Work out the finished part from the listing and answer in its coordinate system (mm). A direction names the side the tool comes from. Round coordinates to 2 decimals unless told otherwise and drop trailing zeros. Loops run counter-clockwise (first coordinate to the right, second up) from the corner with the lowest first, then second, coordinate; pieces in that order, holes last. Notation, with made-up numbers: (-12.5, 35.5) - (28.5, 35.5) arc R10 ccw to (28.5, 51.5) - close; hole circle Ø7 at (78.25, 37). An arc over 180 degrees is marked (long way). Return JSON: item names as keys, results as strings.
from build123d import *

# Parameters (mm, degrees)
SKETCH1_W           = 190
SKETCH1_H           = 140
BOSS_EXTRUDE1_DEPTH = 6
CUT_EXTRUDE1_DEPTH  = 10
SKETCH4_W           = 5
SKETCH4_H           = 140
BOSS_EXTRUDE4_DEPTH = 4
SKETCH8_W           = 190
SKETCH8_H           = 10
BOSS_EXTRUDE8_DEPTH = 10
SKETCH9_W           = 190
SKETCH9_H           = 10
BOSS_EXTRUDE9_DEPTH = 10
SKETCH10_W          = 4
SKETCH10_H          = 8
CUT_EXTRUDE3_DEPTH  = 10
SKETCH11_R          = 3
CUT_EXTRUDE4_DEPTH  = 10
SKETCH12_R          = 4.5
CUT_EXTRUDE6_DEPTH  = 243.148714636
SKETCH3_W           = 150
SKETCH3_H           = 82.5
CUT_EXTRUDE7_DEPTH  = 10
CUT_EXTRUDE9_DEPTH  = 10


with BuildPart() as part:
    # Sketch1 → Boss-Extrude1 (new body)
    with BuildSketch(Plane(origin=(0, 0, 0), x_dir=(1, 0, 0), z_dir=(0, 1, 0))):
        with Locations((95, 70)):
            Rectangle(SKETCH1_W, SKETCH1_H)
    extrude(amount=BOSS_EXTRUDE1_DEPTH)

    # Sketch2 → Cut-Extrude1 (cut)
    with BuildSketch(Plane(origin=(0, 6, 0), x_dir=(1, 0, 0), z_dir=(0, 1, 0))):
        with BuildLine():
            Line((147.071067812, 127.071067812), (112.928932188, 92.928932188))
            ThreePointArc((112.928932188, 92.928932188), (109.6846987, 90.761204675), (105.857864376, 90))
            Line((105.857864376, 90), (0, 90))
            Line((0, 90), (0, 77.5))
            Line((0, 77.5), (94.092172608, 77.5))
            ThreePointArc((94.092172608, 77.5), (95.939931673, 76.265366865), (95.50638617, 74.085786438))
            Line((95.50638617, 74.085786438), (86.849531921, 65.428932188))
            ThreePointArc((86.849531921, 65.428932188), (83.605298432, 63.261204675), (79.778464109, 62.5))
            Line((79.778464109, 62.5), (30.446951372, 62.5))
            Line((30.446951372, 62.5), (0, 62.5))
            Line((0, 62.5), (0, 47.5))
            Line((0, 47.5), (88.357864376, 47.5))
            ThreePointArc((88.357864376, 47.5), (92.1846987, 46.738795325), (95.428932188, 44.571067812))
            Line((95.428932188, 44.571067812), (127.071067812, 12.928932188))
            ThreePointArc((127.071067812, 12.928932188), (130.3153013, 10.761204675), (134.142135624, 10))
            Line((134.142135624, 10), (170, 10))
            ThreePointArc((170, 10), (177.071067812, 12.928932188), (180, 20))
            Line((180, 20), (180, 120))
            ThreePointArc((180, 120), (177.071067812, 127.071067812), (170, 130))
            Line((170, 130), (154.142135624, 130))
            ThreePointArc((154.142135624, 130), (150.3153013, 129.238795325), (147.071067812, 127.071067812))
        make_face()
        with BuildLine():
            Line((94.092172608, 77.5), (0, 77.5))
            Line((0, 77.5), (0, 62.5))
            Line((0, 62.5), (30.446951372, 62.5))
            Line((30.446951372, 62.5), (79.778464109, 62.5))
            ThreePointArc((79.778464109, 62.5), (83.605298432, 63.261204675), (86.849531921, 65.428932188))
            Line((86.849531921, 65.428932188), (95.50638617, 74.085786438))
            ThreePointArc((95.50638617, 74.085786438), (95.939931673, 76.265366865), (94.092172608, 77.5))
        make_face()
    extrude(amount=-CUT_EXTRUDE1_DEPTH, mode=Mode.SUBTRACT)

    # Sketch4 → Boss-Extrude4 (add)
    with BuildSketch(Plane.XZ):
        with Locations((187.5, -70)):
            Rectangle(SKETCH4_W, SKETCH4_H)
    extrude(amount=BOSS_EXTRUDE4_DEPTH)

    # Sketch8 → Boss-Extrude8 (add)
    with BuildSketch(Plane.XY):
        with Locations((95, 1)):
            Rectangle(SKETCH8_W, SKETCH8_H)
    extrude(amount=BOSS_EXTRUDE8_DEPTH)

    # Sketch9 → Boss-Extrude9 (add)
    with BuildSketch(Plane(origin=(0, 0, -140), x_dir=(-1, 0, 0), z_dir=(0, 0, -1))):
        with Locations((-95, 1)):
            Rectangle(SKETCH9_W, SKETCH9_H)
    extrude(amount=BOSS_EXTRUDE9_DEPTH)

    # Sketch10 → Cut-Extrude3 (cut)
    with BuildSketch(Plane.XZ):
        with Locations((2, -16.5)):
            Rectangle(SKETCH10_W, SKETCH10_H)
    extrude(amount=-CUT_EXTRUDE3_DEPTH, mode=Mode.SUBTRACT)

    # Sketch11 → Cut-Extrude4 (cut)
    with BuildSketch(Plane(origin=(0, 6, 0), x_dir=(1, 0, 0), z_dir=(0, 1, 0))):
        with Locations(Location((50, 10, 0), (0, 0, 270))):
            Circle(SKETCH11_R)
        with Locations(Location((110, 10, 0), (0, 0, 270))):
            Circle(SKETCH11_R)
        with Locations(Location((110, 130, 0), (0, 0, 90))):
            Circle(SKETCH11_R)
        with Locations(Location((50, 130, 0), (0, 0, 90))):
            Circle(SKETCH11_R)
    extrude(amount=-CUT_EXTRUDE4_DEPTH, mode=Mode.SUBTRACT)

    # Sketch12 → Cut-Extrude6 (cut, through all)
    with BuildSketch(Plane(origin=(0, 0, 0), x_dir=(1, 0, 0), z_dir=(0, 1, 0))):
        with Locations(Location((50, 10, 0), (0, 0, 270))):
            Circle(SKETCH12_R)
        with Locations(Location((110, 10, 0), (0, 0, 270))):
            Circle(SKETCH12_R)
        with Locations(Location((110, 130, 0), (0, 0, 90))):
            Circle(SKETCH12_R)
        with Locations(Location((50, 130, 0), (0, 0, 90))):
            Circle(SKETCH12_R)
    extrude(amount=CUT_EXTRUDE6_DEPTH, mode=Mode.SUBTRACT)

    # Sketch3 → Cut-Extrude7 (cut)
    with BuildSketch(Plane(origin=(0, 6, 0), x_dir=(1, 0, 0), z_dir=(0, 1, 0))):
        with Locations((75, 71.25)):
            Rectangle(SKETCH3_W, SKETCH3_H)
    extrude(amount=-CUT_EXTRUDE7_DEPTH, mode=Mode.SUBTRACT)

    # Sketch14 → Cut-Extrude9 (cut)
    with BuildSketch(Plane(origin=(0, 6, 0), x_dir=(1, 0, 0), z_dir=(0, 1, 0))):
        with BuildLine():
            Line((127.071067812, 12.928932188), (112.928932188, 27.071067812))
            ThreePointArc((112.928932188, 27.071067812), (109.6846987, 29.238795325), (105.857864376, 30))
            Line((105.857864376, 30), (0, 30))
            Line((0, 30), (0, 112.5))
            Line((0, 112.5), (128.357864376, 112.5))
            ThreePointArc((128.357864376, 112.5), (132.1846987, 113.261204675), (135.428932188, 115.428932188))
            Line((135.428932188, 115.428932188), (147.071067812, 127.071067812))
            Line((147.071067812, 127.071067812), (147.071067812, 92.661701481))
            Line((147.071067812, 92.661701481), (127.071067812, 12.928932188))
        make_face()
    extrude(amount=-CUT_EXTRUDE9_DEPTH, mode=Mode.SUBTRACT)


solid = part.part
1) Section B-B (y = 1.75) is taken. Give the vertices of the cut face in (x, z).
Verdict:
{"outline": "(0, -150) - (190, -150) - (190, 10) - (0, 10) - (0, -12.5) - (4, -12.5) - (4, -20.5) - (0, -20.5) - (0, -30) - (105.86, -30) arc R10 ccw to (112.93, -27.07) - (127.07, -12.93) arc R10 cw to (134.14, -10) - (170, -10) arc R10 cw to (180, -20) - (180, -120) arc R10 cw to (170, -130) - (154.14, -130) arc R10 cw to (147.07, -127.07) - (135.43, -115.43) arc R10 ccw to (128.36, -112.5) - (0, -112.5) - close; hole circle Ø9 at (50, -130); hole circle Ø9 at (50, -10); hole circle Ø9 at (110, -130); hole circle Ø9 at (110, -10)"}
2) Section D-D (x = 50) is taken. Give the vertices of the cut face in (y, z).
Verdict:
{"outline": "(-4, -150) - (6, -150) - (6, -134.5) - (0, -134.5) - (0, -140) - (-4, -140) - close; (-4, 0) - (0, 0) - (0, -5.5) - (6, -5.5) - (6, 10) - (-4, 10) - close; (0, -125.5) - (6, -125.5) - (6, -112.5) - (0, -112.5) - close; (0, -30) - (6, -30) - (6, -14.5) - (0, -14.5) - close"}
3) Section C-C (z = -122) is taken. Give the vertices of the cut face in (x, y).
Verdict:
{"outline": "(0, 0) - (142, 0) - (142, 6) - (0, 6) - close; (179.8, 0) - (185, 0) - (185, -4) - (190, -4) - (190, 6) - (179.8, 6) - close"}
4) Find the intervals of material crossed by L1, parallel to Z at x = 50, y = 2.2; L2, parallel to Z at x = 88.5, y = 2.75; L3, parallel to Z at x = 168.5, y = 4.25, in increasing order.
Verdict:
{"L1": "z = -150 to -134.5, -125.5 to -112.5, -30 to -14.5, -5.5 to 10", "L2": "z = -150 to -112.5, -30 to 10", "L3": "z = -150 to -130, -10 to 10"}
5) Determine the mould class of faces 4 (the flat face through (94, 1, 10)), 5 (the flat face through (185, -2, -71)), 6 (the cylindrical face through (150.37, 3.04, -129.26)) for opening direction X: pulls with the +X half, pulls with the -X half, needs draft (parallel to the pull), parting line crosses it, or undercut.
Verdict:
{"face 4": "needs draft", "face 5": "pulls with the -X half", "face 6": "undercut"}
6) Section A-A (x = 24.5) is taken. Give the vertices of the cut face in (y, z).
Verdict:
{"outline": "(-4, -150) - (6, -150) - (6, -112.5) - (0, -112.5) - (0, -140) - (-4, -140) - close; (-4, 0) - (0, 0) - (0, -30) - (6, -30) - (6, 10) - (-4, 10) - close"}
7) Flat-ended cylindrical pins translate along their axes: pin 1 (10 mm diameter, centred on x = 148.5, z = -7, fed in from -Y); pin 2 (3 mm diameter, centred on y = 2, z = -64, fed in from -X). Find the tip coordinate at first contact, or state that the pin passes through.
Verdict:
{"pin 1": "stops at y = 0", "pin 2": "stops at x = 180"}
8) A tool of negligible diameter and unlimited length cuts with its end or side. For faces 1 (the flat face through (2, 3, -12.5)), 2 (the cylindrical face through (177.15, 3.04, -126.99)), 3 (the flat face through (91, -2, 0)), from which of +Z, -Z, +X, -X, +Y, -Y can it reach the whole face along a straight path? Write none if from no direction.
Verdict:
{"face 1": "-X, +Y, -Y", "face 2": "+Y, -Y", "face 3": "-X, -Y"}
